Geometry: final body of the model. Coordinates: model frame, mm. Face numbers are marked on the shaded views. A direction names the side the tool comes from. Round coordinates to 2 decimals unless told otherwise and drop trailing zeros. Write each loop counter-clockwise with the first axis right and the second up, starting at its lowest first coordinate (ties: lowest second). Pieces come first, ordered by that corner, then holes. Notation, with made-up numbers: (-1.75, 38) -> (13.25, 38) arc R25 cw to (13.25, 76) -> close; hole circle Ø1 at (13.25, 43). An arc over 180 degrees is marked (long way). One line per item, written item: value. Start each with the question number.
Autodesk Inventor part; units mm, degrees
ref_plane "YZ Plane" through (0, 0, 0) normal (1, 0, 0) x (0, 1, 0)
ref_plane "XZ Plane" through (0, 0, 0) normal (0, 1, 0) x (-1, 0, 0)
ref_plane "XY Plane" through (0, 0, 0) normal (0, 0, 1) x (1, 0, 0)
sketch "Sketch1" plane through (0, 0, 0) normal (0, 1, 0) x (-1, 0, 0)
  line L0 (55, 25) -> (-55, 25)
  line L1 (-55, 25) -> (-55, -25)
  line L2 (-55, -25) -> (55, -25)
  line L3 (55, -25) -> (55, 25)
  line L4 (55, 25) -> (-55, -25) construction
  line L5 (-55, 25) -> (55, -25) construction
  line L6 (-25, 25) -> (25, 25)
  line L7 (25, 25) -> (25, -25)
  line L8 (25, -25) -> (-25, -25)
  line L9 (-25, -25) -> (-25, 25)
  line L10 (-25, 25) -> (25, -25) construction
  line L11 (25, 25) -> (-25, -25) construction
  point P0 (0, 0)
  dimension "d0" = 110
  dimension "d1" = 50
  dimension "d2" = 50
  dimension "d3" = 50
extrude "Extrusion1" add sketch "Sketch1" along normal blind 10 contours L3 L2 L7 L0 | L9 L2 L1 L0
sketch "Sketch2" plane through (0, 10, 0) normal (0, 1, 0) x (1, 0, 0)
  line L0 (-35, -25) -> (-25, -25)
  line L1 (-25, -25) -> (-25, 25)
  line L2 (-25, 25) -> (-35, 25)
  line L3 (-35, 25) -> (-35, -25)
  line L4 (-35, -25) -> (-25, 25) construction
  line L5 (-25, -25) -> (-35, 25) construction
  line L6 (25, -25) -> (35, -25)
  line L7 (35, -25) -> (35, 25)
  line L8 (35, 25) -> (25, 25)
  line L9 (25, 25) -> (25, -25)
  line L10 (25, -25) -> (35, 25) construction
  line L11 (35, -25) -> (25, 25) construction
  line L12 (-25, -25) -> (-25, 25)
  line L13 (25, 25) -> (25, -25)
  point P0 (0, 0)
  point P1 (-30, 0)
  point P2 (30, 0)
  dimension "d6" = 10
  dimension "d7" = 50
  dimension "d8" = 10
  dimension "d9" = 50
extrude "Extrusion2" add sketch "Sketch2" along normal blind 40
sketch "Sketch3" plane through (0, 50, 0) normal (0, 1, 0) x (1, 0, 0)
  line L0 (-25, -25) -> (25, -25)
  line L1 (25, -25) -> (25, 25)
  line L2 (25, 25) -> (-25, 25)
  line L3 (-25, 25) -> (-25, -25)
  line L4 (-25, -25) -> (25, 25) construction
  line L5 (25, -25) -> (-25, 25) construction
  line L6 (25, 25) -> (25, -25)
  line L7 (35, 25) -> (25, 25)
  point P0 (0, 0)
extrude "Extrusion3" add sketch "Sketch3" against normal blind 5
sketch "Sketch4" plane through (0, 50, 0) normal (0, 1, 0) x (1, 0, 0)
  circle A0 centre (0, 0) radius 9.75
  dimension "d14" = 19.5
extrude "Extrusion4" cut sketch "Sketch4" against normal blind 5
sketch "Sketch5" plane through (0, 10, 0) normal (0, 1, 0) x (1, 0, 0)
  circle A0 centre (-45, 0) radius 3.05
  circle A1 centre (45, 0) radius 3.05
  line L0 (55, -25) -> (55, 25)
  line L1 (-55, 25) -> (-55, -25)
  point P0 (0, 0)
  dimension "d17" = 6.1
  dimension "d18" = 6.1
  dimension "d22" = 10
  dimension "d23" = 10
extrude "Extrusion5" cut sketch "Sketch5" against normal through all
fillet "Fillet1" radius 2 28 edges at (-55, 10, 0) (-35, 10, 0) (-35, 50, 0) (35, 50, 0) (35, 10, 0) (55, 10, 0) (45, 10, 25) (45, 10, -25) (55, 5, 25) (55, 5, -25) (-45, 10, 25) (-55, 5, 25) (-55, 5, -25) (-45, 10, -25) (35, 30, 25) (35, 30, -25) (0, 50, -25) (0, 50, 25) (-35, 30, 25) (-35, 30, -25) (-25, 22.5, -25) (-25, 22.5, 25) (25, 22.5, -25) (25, 22.5, 25) (0, 45, 25) (0, 45, -25) (-25, 45, 0) (25, 45, 0)
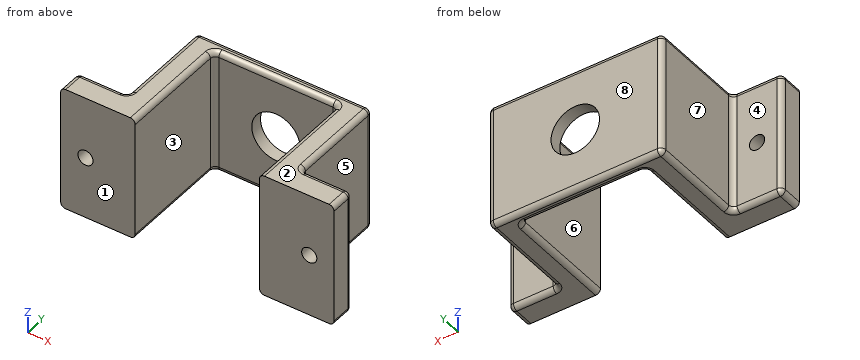
(1) Pull-direction query (X, two-part tool) for the marked faces 6, 7 and 8; classes: pulls with the +X half, pulls with the -X half, needs draft (parallel to the pull), parting line crosses it, or undercut.
(2) Section query D-D (z = 5.5). Output: boundary loops of the cut face in (x, y).
(3) Section query C-C (y = 26). Output: boundary loops of the cut face in (x, z), and give its area (3 significant figures).
(4) Line query: probe 1 along X at (y, z) = (2.25, 0); probe 2 along Z at (x, y) = (0, 48.25); probe 3 along Z at (x, y) = (45, 2). Output: solid intervals per line, ascending.
(5) Set-up query: the marked faces 1, 2, 3, 4 and 5. Return all of +Z, -Z, +X, -X, +Y, -Y with unobstructed straight access to the full face (end or side cutting, diameter ignored); none if empty.
(6) Section query A-A (x = -45). Output: boundary loops of the cut face in (y, z).
(7) Section query B-B (z = 0). Count the separate pieces of the cut face and the enclosed holes in it, and give its area (3 significant figures).
(8) Pin query (flat end, axial travel): pin 1 (5 mm diameter, centred on y = 23.5, z = -3, fed in from -X); pin 2 (5.5 mm diameter, centred on x = -45, z = 0, fed in from +Y) (1 decimal); pin 3 (8 mm diameter, centred on x = 43, z = -5.5, fed in from +Y); pin 4 (3 mm diameter, centred on x = -16, z = 7.5, fed in from -Y). Return the tip coordinate at first contact, or that it passes through.
Results list:
1. face 6: undercut
1. face 7: pulls with the -X half
1. face 8: needs draft
2. outline: (-55, 0) -> (-25, 0) -> (-25, 43) arc R2 cw to (-23, 45) -> (-8.05, 45) -> (-8.05, 50) -> (-33, 50) arc R2 ccw to (-35, 48) -> (-35, 12) arc R2 cw to (-37, 10) -> (-53, 10) arc R2 ccw to (-55, 8) -> close; (8.05, 45) -> (23, 45) arc R2 cw to (25, 43) -> (25, 0) -> (55, 0) -> (55, 8) arc R2 ccw to (53, 10) -> (37, 10) arc R2 cw to (35, 12) -> (35, 48) arc R2 ccw to (33, 50) -> (8.05, 50) -> close
3. outline: (-35, -23) arc R2 ccw to (-33, -25) -> (-27, -25) arc R2 ccw to (-25, -23) -> (-25, 23) arc R2 ccw to (-27, 25) -> (-33, 25) arc R2 ccw to (-35, 23) -> close; (25, -23) arc R2 ccw to (27, -25) -> (33, -25) arc R2 ccw to (35, -23) -> (35, 23) arc R2 ccw to (33, 25) -> (27, 25) arc R2 ccw to (25, 23) -> close
3. area: 993 mm^2
4. probe 1: x = -55 to -48.05, -41.95 to -25, 25 to 41.95, 48.05 to 55
4. probe 2: z = -24.98 to -9.75, 9.75 to 24.98
4. probe 3: z = -25 to -3.05, 3.05 to 25
5. face 1: +Z, -Z, +X, -X, -Y
5. face 2: +Z, +X, -X, +Y, -Y
5. face 3: +Z, -Z, -Y
5. face 4: +Z, -Z, -X, +Y
5. face 5: +Z, -Z, +X, +Y
6. outline: (0, -25) -> (8, -25) arc R2 ccw to (10, -23) -> (10, -3.05) -> (0, -3.05) -> close; (0, 3.05) -> (10, 3.05) -> (10, 23) arc R2 ccw to (8, 25) -> (0, 25) -> close
7. separate pieces: 4
7. enclosed holes: 0
7. area: 1,430 mm^2
8. pin 1: stops at x = -35
8. pin 2: passes through
8. pin 3: stops at y = 10
8. pin 4: stops at y = 45
